Source: three-view drawing plus pictorial views. Frame: mm from the lowest corner of the part. Give positions to 0.01 mm unless a question says otherwise; leave off trailing zeros. Loops run counter-clockwise (first coordinate to the right, second up) from the corner with the lowest first, then second, coordinate; pieces in that order, holes last. Notation, with made-up numbers: (23.5, 81) - (64.5, 81) arc R13 cw to (64.5, 93) - close; hole circle Ø1 at (-7, -7). An arc over 180 degrees is marked (long way). Write each question's results on one line, items separated by ' | '. Start each with the question number.
(1) Cut plane D-D on x = 81.5. Return the cut outline in (y, z) (1 decimal).
(2) Cut plane C-C on z = 33. Give the number of separate pieces and of enclosed holes in the cut face, then the cut area to 3 significant figures.
(3) Cut plane A-A on y = 49. Return the cut outline in (x, z) (1 decimal).
(4) Material intervals for line 1 along Z through (x, y) = (20, 54); line 2 along Y through (x, z) = (117.5, 16) (1 decimal); line 3 along Z through (x, y) = (40, 61), sorted ascending. Write a range as [from, to].
(5) Contact query for flat-ended pins moving along their axis: pin 1 (8.5 mm diameter, centred on x = 100, z = 8, fed in from +Y); pin 2 (8 mm diameter, centred on y = 18, z = 42, fed in from +X) (1 decimal); pin 3 (3 mm diameter, centred on y = 14, z = 31.5, fed in from -X); pin 4 (2 mm diameter, centred on x = 109, y = 62.5, fed in from -Z). Output: stop coordinate, or through.
(6) Pull-direction query (X, two-part tool) for the marked faces 1, 2 and 3; classes: pulls with the +X half, pulls with the -X half, needs draft (parallel to the pull), parting line crosses it, or undercut.
(7) Cut plane B-B on x = 58. Return the cut outline in (y, z) (1 decimal).
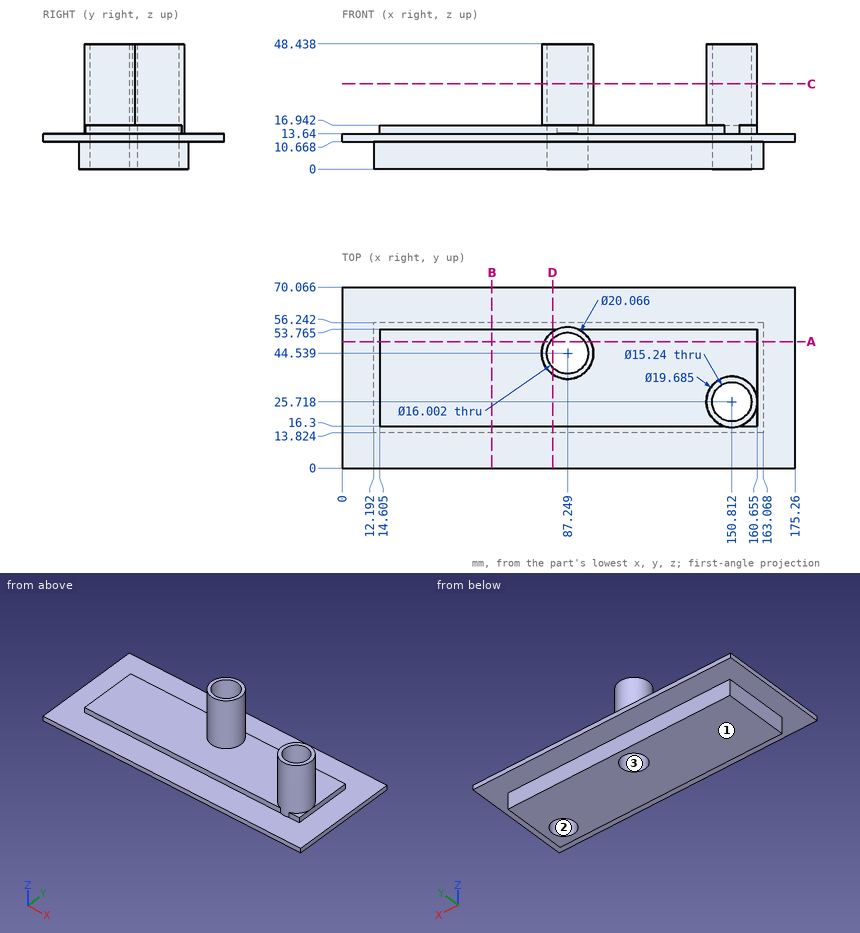
Ans:
1) outline: (0, 10.7) - (13.8, 10.7) - (13.8, 0) - (39, 0) - (39, 48.4) - (36.3, 48.4) - (36.3, 16.9) - (16.3, 16.9) - (16.3, 13.6) - (0, 13.6) - close; (50.1, 0) - (56.2, 0) - (56.2, 10.7) - (70.1, 10.7) - (70.1, 13.6) - (53.8, 13.6) - (53.8, 16.9) - (52.8, 16.9) - (52.8, 48.4) - (50.1, 48.4) - close
2) separate pieces: 2 | enclosed holes: 2 | area: 237 mm^2
3) outline: (0, 10.7) - (12.2, 10.7) - (12.2, 0) - (80.6, 0) - (80.6, 48.4) - (78.3, 48.4) - (78.3, 16.9) - (14.6, 16.9) - (14.6, 13.6) - (0, 13.6) - close; (93.9, 0) - (163.1, 0) - (163.1, 10.7) - (175.3, 10.7) - (175.3, 13.6) - (160.7, 13.6) - (160.7, 16.9) - (96.2, 16.9) - (96.2, 48.4) - (93.9, 48.4) - close
4) line 1: [0, 13.64] | line 2: [16.3, 53.8] | line 3: [10.67, 13.64]
5) pin 1: y = 70.07 | pin 2: x = 159.9 | pin 3: through | pin 4: z = 10.67
6) face 1: needs draft | face 2: undercut | face 3: undercut
7) outline: (0, 10.7) - (13.8, 10.7) - (13.8, 0) - (56.2, 0) - (56.2, 10.7) - (70.1, 10.7) - (70.1, 13.6) - (53.8, 13.6) - (53.8, 16.9) - (16.3, 16.9) - (16.3, 13.6) - (0, 13.6) - close
